```python
from build123d import *

# Parameters (mm, degrees)
F0_R      = 9.4996
F1_DEPTH  = 5.461
F2_R      = 2.794
F3_DEPTH  = 12.0396
F4_R      = 2.8321
F5_DEPTH  = 3.3782
F6_R      = 2.0955
F7_DEPTH  = 4.445
F8_R      = 1.6002
F9_DEPTH  = 25.4
F10_DEPTH = 7.2136


with BuildPart() as f1:
    # F0 (on Top) → F1 (new body)
    with BuildSketch(Plane.XY):
        Circle(F0_R)
    extrude(amount=F1_DEPTH)

    # F2 (on face) → F3 (join)
    with BuildSketch(Plane.XY.offset(5.461)):
        Circle(F2_R)
    extrude(amount=F3_DEPTH)

    # F4 (on face) → F5 (cut)
    with BuildSketch(Plane.XY.offset(5.461)):
        with Locations((-5.8801, 0)):
            Circle(F4_R)
        with Locations((5.8801, 0)):
            Circle(F4_R)
    extrude(amount=-F5_DEPTH, mode=Mode.SUBTRACT)

    # F6 (on face) → F7 (cut)
    with BuildSketch(Plane(origin=(0, 0, 0), x_dir=(1, 0, 0), z_dir=(0, 0, -1))):
        Circle(F6_R)
    extrude(amount=-F7_DEPTH, mode=Mode.SUBTRACT)

    # F8 (on face) → F9 (cut)
    with BuildSketch(Plane(origin=(0, 0, 0), x_dir=(1, 0, 0), z_dir=(0, 0, -1))):
        with Locations((5.969, 0)):
            Circle(F8_R)
        with Locations((-5.969, 0)):
            Circle(F8_R)
    extrude(amount=-F9_DEPTH, mode=Mode.SUBTRACT)

    # F10 (add): a face of the model
    f10_faces = [f1.faces().sort_by_distance(p)[0] for p in [
        (-9.2309107369, 0, 5.461),
    ]]
    extrude(f10_faces, amount=F10_DEPTH)


solid = f1.part
```
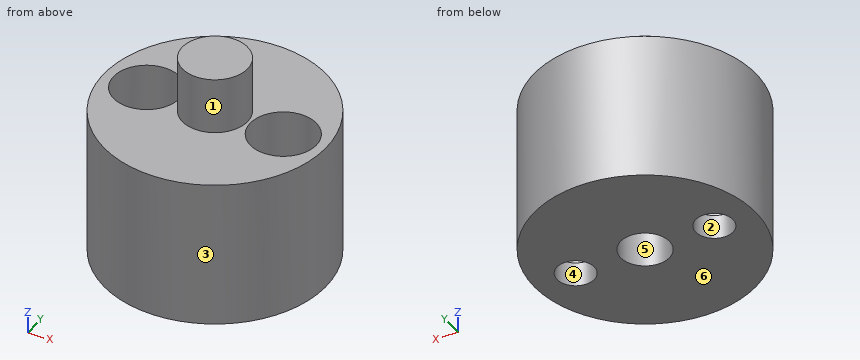
The listing builds one solid part. Answer for the finished solid, in the listing's coordinates (mm). Face numbers are marked on the shaded views. A direction names the side the tool comes from. Give positions to 0.01 mm unless a question says otherwise; leave off trailing zeros. Loops run counter-clockwise (first coordinate to the right, second up) from the corner with the lowest first, then second, coordinate; pieces in that order, holes last. Notation, with made-up numbers: (-23, -25.5) - (31, -25.5) arc R21 cw to (31, 11.5) - close; hole circle Ø2 at (39.25, -11). An arc over 180 degrees is marked (long way). Return JSON: item names as keys, results as strings. Group by question number.
1. Straight lines are drawn through the part: line 1 (Y direction, x = 0, z = 2); line 2 (X direction, y = -0.5, z = 8); line 3 (Z direction, x = -5.75, y = -3.5). For each, find the intervals that lie inside material, in ascending order. Write a range as [from, to].
2. Determine the mould class of the marked faces 3, 4, 5 and 6 for opening direction Y: pulls with the +Y half, pulls with the -Y half, needs draft (parallel to the pull), parting line crosses it, or undercut.
3. Given pin 1 Ø1.7 at (x, y) = (6.5, -1.5) entering from +Z; pin 2 Ø1 at (x, z) = (-1.5, 2) entering from -Y; pin 3 Ø4.5 at (x, y) = (-6.5, 0.5) entering from +Z, each flat-ended and moving along its own axis, determine where each tip first touches the part or whether it passes through.
4. Which of the six approach directions +Z, -Z, +X, -X, +Y, -Y give full straight-line access (tool end or side, diameter ignored) to the marked faces 1 and 2?
5. Find section A-A (y = 0). State how many separate pieces and enclosed holes the cut face has, then the cut area to 3 significant figures.
6. Find section D-D (x = 6.25). Write down the section's boundary in (y, z).
7. Find section C-C (z = 3.75). Write down the section's boundary in (x, y).
8. Find section B-B (x = 0). Write down the section's boundary in (y, z) (1 decimal), then the cut area to 3 significant figures.
Verdict:
{
 "1": {"line 1": "y = [-9.5, -2.1], [2.1, 9.5]", "line 2": "x = [-9.49, -8.67], [-3.09, 3.09], [8.67, 9.49]", "line 3": "z = [0, 12.67]"},
 "2": {"face 3": "parting line crosses it", "face 4": "undercut", "face 5": "undercut", "face 6": "needs draft"},
 "3": {"pin 1": "stops at z = 2.08", "pin 2": "stops at y = -9.45", "pin 3": "stops at z = 12.67"},
 "4": {"face 1": "+Z", "face 2": "+Z, -Z"},
 "5": {"separate pieces": "3", "enclosed holes": "0", "area": "116 mm^2"},
 "6": {"outline": "(-7.15, 0) - (-1.58, 0) - (-1.58, 2.08) - (-2.81, 2.08) - (-2.81, 12.67) - (-7.15, 12.67) - close; (1.58, 0) - (7.15, 0) - (7.15, 12.67) - (2.81, 12.67) - (2.81, 2.08) - (1.58, 2.08) - close"},
 "7": {"outline": "circle Ø19 at (0, 0); hole circle Ø5.66 at (-5.88, 0); hole circle Ø4.19 at (0, 0); hole circle Ø5.66 at (5.88, 0)"},
 "8": {"outline": "(-9.5, 0) - (-2.1, 0) - (-2.1, 4.4) - (2.1, 4.4) - (2.1, 0) - (9.5, 0) - (9.5, 12.7) - (2.8, 12.7) - (2.8, 17.5) - (-2.8, 17.5) - (-2.8, 12.7) - (-9.5, 12.7) - close", "area": "249 mm^2"}
}
